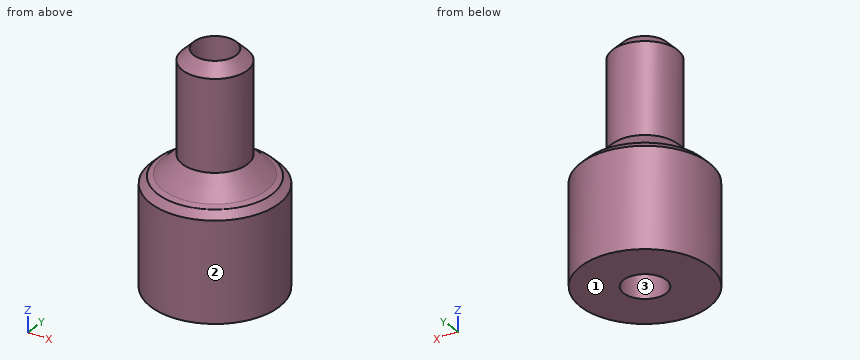
from build123d import *

# Parameters (mm, degrees)
F0_R     = 12.05
F0_R_2   = 4
F1_DEPTH = 45
F2_R     = 13.7736211886
F2_R_2   = 6.1
F3_DEPTH = 25


# Not quite as in the source:
# - a fillet or chamfer that OpenCascade refuses, or shapes differently, is made with other operations: its cross-section is extruded or revolved along the edge and cut away or added


with BuildPart() as f1:
    # F0 (on Top) → F1 (new body)
    with BuildSketch(Plane.XY):
        Circle(F0_R)
        Circle(F0_R_2, mode=Mode.SUBTRACT)
    extrude(amount=F1_DEPTH)

    # F2 (on face) → F3 (cut)
    with BuildSketch(Plane.XY.offset(45)):
        Circle(F2_R)
        Circle(F2_R_2, mode=Mode.SUBTRACT)
    extrude(amount=-F3_DEPTH, mode=Mode.SUBTRACT)

    # F4: chamfer of 4 on 3 edges, made by hand

    # F4_s1 → F4_t2 (revolve)
    with BuildSketch(Plane.XZ):
        Polygon((10.1, 20), (6.1, 24), (6.1, 20), align=None)
    revolve(axis=Axis((0, 0, 20), (0, 0, 1)))

    # F4_s3 → F4_t4 (revolve, cut)
    with BuildSketch(Plane.XZ):
        Polygon((2.1, 45), (6.1, 41), (6.1, 45), align=None)
    revolve(axis=Axis((0, 0, 45), (0, 0, 1)), mode=Mode.SUBTRACT)

    # F5: chamfer of 1.3 on 2 edges, made by hand

    # F5_s1 → F5_t2 (revolve)
    with BuildSketch(Plane.XZ):
        Polygon((10.6384776311, 20), (9.7192388155, 20.3807611845), (10.1, 20), align=None)
    revolve(axis=Axis((0, 0, 20), (0, 0, 1)))

    # F5_s3 → F5_t4 (revolve, cut)
    with BuildSketch(Plane.XZ):
        Polygon((12.05, 18.7), (10.75, 20), (12.05, 20), align=None)
    revolve(axis=Axis((0, 0, 20), (0, 0, -1)), mode=Mode.SUBTRACT)


solid = f1.part
Read the model definition and answer for the solid it produces. Units are mm, in the model's axes. Face numbers are marked on the shaded views. Round coordinates to 2 decimals unless told otherwise and drop trailing zeros. Order: outer loops, then holes, each group sorted by start corner. A loop starts at its lowest first (then second) coordinate and runs counter-clockwise, first axis right, second up.
1) The part is cut by section A-A on y = 0. Write down the section's boundary in (x, z), plus the area to 3 significant figures.
2) Straight lines are drawn through the part: L1, parallel to Y at x = 0, z = 13.5; L2, parallel to Y at x = 0, z = 26. For each, find the intervals that lie inside material, in ascending order.
3) Flat-ended cylindrical pins translate along their axes: pin 1 (3 mm diameter, centred on y = 2.5, z = 7.5, fed in from +X); pin 2 (10 mm diameter, centred on x = -2, y = 9.5, fed in from +Z); pin 3 (1.5 mm diameter, centred on x = 6, y = 5, fed in from +Z). Find the tip coordinate at first contact, or state that the pin passes through.
4) The part is cut by section D-D on z = 39. Write down the section's boundary in (x, y).
5) The mould has two halves that part along X. Classify the marked faces 1, 2 and 3: released by +X, released by -X, zero draft, split by the parting line, or undercut.
6) The part is cut by section C-C on z = 10. Write down the section's boundary in (x, y), plus the area to 3 significant figures.
Resolved:
1. outline: (-12.05, 0) - (-4, 0) - (-4, 43.1) - (-6.1, 41) - (-6.1, 24) - (-9.72, 20.38) - (-10.64, 20) - (-10.75, 20) - (-12.05, 18.7) - close; (4, 0) - (12.05, 0) - (12.05, 18.7) - (10.75, 20) - (10.64, 20) - (9.72, 20.38) - (6.1, 24) - (6.1, 41) - (4, 43.1) - close
1. area: 429 mm2
2. L1: y = -12.05 to -4, 4 to 12.05
2. L2: y = -6.1 to -4, 4 to 6.1
3. pin 1: stops at x = 12.01
3. pin 2: stops at z = 42.39
3. pin 3: stops at z = 23.04
4. outline: circle Ø12.2 at (0, 0); hole circle Ø8 at (0, 0)
5. face 1: zero draft
5. face 2: split by the parting line
5. face 3: undercut
6. outline: circle Ø24.1 at (0, 0); hole circle Ø8 at (0, 0)
6. area: 406 mm2
